Autodesk Inventor part; units mm, degrees
ref_plane "YZ Plane" through (0, 0, 0) normal (1, 0, 0) x (0, 1, 0)
ref_plane "XZ Plane" through (0, 0, 0) normal (0, 1, 0) x (-1, 0, 0)
ref_plane "XY Plane" through (0, 0, 0) normal (0, 0, 1) x (1, 0, 0)
sketch "Sketch1" plane through (0, 0, 0) normal (0, 1, 0) x (-1, 0, 0)
  line L0 (-40, 40) -> (40, 40)
  line L1 (40, 40) -> (40, -40)
  line L2 (40, -40) -> (-40, -40)
  line L3 (-40, -40) -> (-40, 40)
  line L4 (-40, 40) -> (40, -40) construction
  line L5 (40, 40) -> (-40, -40) construction
  line L6 (-25, 25) -> (25, 25) construction
  line L7 (25, 25) -> (25, -25) construction
  line L8 (25, -25) -> (-25, -25) construction
  line L9 (-25, -25) -> (-25, 25) construction
  line L10 (-25, 25) -> (25, -25) construction
  line L11 (25, 25) -> (-25, -25) construction
  line L12 (-20, 25) -> (20, 25) construction
  line L13 (20, 25) -> (20, -25) construction
  line L14 (20, -25) -> (-20, -25) construction
  line L15 (-20, -25) -> (-20, 25) construction
  line L16 (-20, 25) -> (20, -25) construction
  line L17 (20, 25) -> (-20, -25) construction
  circle A0 centre (0, 0) radius 10
  dimension "d0" = 80
  dimension "d1" = 50
  dimension "d2" = 40
  dimension "d3" = 20
extrude "Extrusion1" add sketch "Sketch1" against normal blind 10
hole "Hole1" at (-20, 0, -25) at (20, 0, -25) at (-25, 0, 25) at (25, 0, 25) direction (0, -1, 0) diameter 10.5 end through all
chamfer "Chamfer1" distance 0.5 angle 45 10 edges at (20, 0, -30.25) (-20, 0, -30.25) (25, 0, 19.75) (-25, 0, 19.75) (20, -10, -30.25) (-20, -10, -30.25) (25, -10, 19.75) (-25, -10, 19.75) (10, 0, 0) (10, -10, 0)
properties part number "AP1-002"
Read the model definition and answer for the solid it produces. Units are mm, in the model's axes. Give positions to 0.01 mm unless a question says otherwise; leave off trailing zeros. Order: outer loops, then holes, each group sorted by start corner. A loop starts at its lowest first (then second) coordinate and runs counter-clockwise, first axis right, second up.
(1) For a pull along Z with two mould halves and no side action, classify faces 1 (the cylindrical face through (-20.231, -5.063, -30.245)), 2 (the flat face through (-8, -10, 9)), 3 (the flat face through (-1, -5, -40)) as released by +Z, released by -Z, zero draft, split by the parting line, or undercut.
(2) Find section A-A (z = -25). Give the vertices of the cut face in (x, y).
(3) Find section C-C (z = 0). Give the vertices of the cut face in (x, y), plus the area to 4 significant figures.
(4) Find section B-B (y = -7.75). Give the vertices of the cut face in (x, z).
(5) Straight lines are drawn through the part: L1, parallel to X at y = -7.25, z = -25; L2, parallel to X at y = -8.5, z = 25; L3, parallel to Z at x = 22.5, y = -4. For each, find the intervals that lie inside material, in ascending order.
Result sheet:
1. face 1: undercut
1. face 2: zero draft
1. face 3: released by -Z
2. outline: (-40, -10) - (-25.75, -10) - (-25.25, -9.5) - (-25.25, -0.5) - (-25.75, 0) - (-40, 0) - close; (-14.75, -9.5) - (-14.25, -10) - (14.25, -10) - (14.75, -9.5) - (14.75, -0.5) - (14.25, 0) - (-14.25, 0) - (-14.75, -0.5) - close; (25.25, -9.5) - (25.75, -10) - (40, -10) - (40, 0) - (25.75, 0) - (25.25, -0.5) - close
3. outline: (-40, -10) - (-10.5, -10) - (-10, -9.5) - (-10, -0.5) - (-10.5, 0) - (-40, 0) - close; (10, -9.5) - (10.5, -10) - (40, -10) - (40, 0) - (10.5, 0) - (10, -0.5) - close
3. area: 599.5 mm2
4. outline: (-40, -40) - (40, -40) - (40, 40) - (-40, 40) - close; hole circle Ø10.5 at (-25, 25); hole circle Ø10.5 at (-20, -25); hole circle Ø20 at (0, 0); hole circle Ø10.5 at (20, -25); hole circle Ø10.5 at (25, 25)
5. L1: x = -40 to -25.25, -14.75 to 14.75, 25.25 to 40
5. L2: x = -40 to -30.25, -19.75 to 19.75, 30.25 to 40
5. L3: z = -40 to -29.62, -20.38 to 20.38, 29.62 to 40
